For this review, take the finished solid that the model builds, in its own axes (mm). A direction names the side the tool comes from. Round coordinates to 2 decimals unless told otherwise and drop trailing zeros. Order: outer loops, then holes, each group sorted by start corner. A loop starts at its lowest first (then second) coordinate and runs counter-clockwise, first axis right, second up.
from build123d import *

# Parameters (mm, degrees)
SKETCH1_R           = 1.5
BOSS_EXTRUDE1_DEPTH = 2.3
SKETCH2_R           = 5.65
BOSS_EXTRUDE2_DEPTH = 7.7
BOSS_EXTRUDE3_DEPTH = 26.3
SKETCH5_R           = 1
BOSS_EXTRUDE4_DEPTH = 5.5


with BuildPart() as part:
    # Sketch1 → Boss-Extrude1 (new body)
    with BuildSketch(Plane(origin=(0, 0, 0), x_dir=(1, 0, 0), z_dir=(0, 1, 0))):
        with BuildLine():
            Line((-3, 5.765), (3, 5.765))
            Line((3, 5.765), (10.043565082, 3.861472766))
            ThreePointArc((10.043565082, 3.861472766), (13, 0), (10.043565082, -3.861472766))
            Line((10.043565082, -3.861472766), (3, -5.765))
            Line((3, -5.765), (-3, -5.765))
            Line((-3, -5.765), (-10.043565082, -3.861472766))
            ThreePointArc((-10.043565082, -3.861472766), (-13, 0), (-10.043565082, 3.861472766))
            Line((-10.043565082, 3.861472766), (-3, 5.765))
        make_face()
        with Locations((9, 0)):
            Circle(SKETCH1_R, mode=Mode.SUBTRACT)
        with Locations((-9, 0)):
            Circle(SKETCH1_R, mode=Mode.SUBTRACT)
    extrude(amount=-BOSS_EXTRUDE1_DEPTH)

    # Sketch2 → Boss-Extrude2 (add)
    with BuildSketch(Plane.XZ.offset(2.3)):
        Circle(SKETCH2_R)
    extrude(amount=BOSS_EXTRUDE2_DEPTH)

    # Sketch3 → Boss-Extrude3 (add)
    with BuildSketch(Plane.XZ.offset(10)):
        Polygon((-4, 5.765), (4, 5.765), (6.5, 2.765), (6.5, -5.235), (-6.5, -5.235), (-6.5, 2.765), align=None)
    extrude(amount=BOSS_EXTRUDE3_DEPTH)

    # Sketch4 → Cut-Revolve1 (revolve, cut)
    with BuildSketch(Plane.XY):
        Polygon((3.5, -36.3), (10, -29.8), (10, -36.3), align=None)
    revolve(axis=Axis((0, -36.3, 0), (0, 1, 0)), mode=Mode.SUBTRACT)

    # Sketch5 → Boss-Extrude4 (add)
    with BuildSketch(Plane.XZ.offset(36.3)):
        Circle(SKETCH5_R)
    extrude(amount=BOSS_EXTRUDE4_DEPTH)


solid = part.part
(1) Clearance check with flat-ended pins moving along their axes: P1, Ø14.5, axis at x = 0, y = -21, coming from the -Z side (3 decimals); P2, Ø5, axis at y = -29, z = -3.5, coming from the +X side; P3, Ø2.5, axis at y = -17, z = -2.5, coming from the -X side. State where each tip first meets the part, or that it passes through.
(2) Wall thickness on L1, parallel to Z at x = -2.5, y = -22 (3 decimals); L2, parallel to Y at x = -1.75, z = 5.5; L3, parallel to Y at x = -6.75, z = 3: over which ranges is each line inside the solid? List them lowest first.
(3) Add section B-B on x = 0. Give the boundary of the cut face in (y, z) (3 decimals).
(4) Add section C-C on x = 9. Give the boundary of the cut face in (y, z), plus the area to 3 significant figures.
(5) Tool access review of faces 5 (the face through (0, -39, -1)), 6 (the face through (-6.57, -1.13, -4.8)), 7 (the face through (5.23, -21.36, 4.29)): name each direction out of +Z, -Z, +X, -X, +Y, -Y from which nothing blocks a thin tool from reaching the whole face with its end or side.
(6) Add section A-A on z = 0. Give the boundary of the cut face in (x, y).
(7) Draft analysis for pull direction Y (two halves, no side actions). For faces 1 (the face through (0, -41.8, 0)), 2 (the face through (5.39, -6.1, 1.7)), 3 (the face through (-6.5, -21, -1)), 4 (the face through (5, -10, 3)), state which applies: pulls with the +Y half, pulls with the -Y half, needs draft (parallel to the pull), parting line crosses it, or undercut.
(8) Add section D-D on y = -18. Give the boundary of the cut face in (x, z) (3 decimals), plus the area to 4 significant figures.
Here are the results:
1. P1: stops at z = -5.235
1. P2: stops at x = 6.5
1. P3: stops at x = -6.5
2. L1: z = -5.235 to 5.765
2. L2: y = -34.03 to -10, -2.3 to 0
2. L3: y = -2.3 to 0
3. outline: (-41.8, -1) - (-36.3, -1) - (-36.3, -3.5) - (-34.565, -5.235) - (-10, -5.235) - (-10, -5.65) - (-2.3, -5.65) - (-2.3, -5.765) - (0, -5.765) - (0, 5.765) - (-2.3, 5.765) - (-2.3, 5.65) - (-10, 5.65) - (-10, 5.765) - (-34.035, 5.765) - (-36.3, 3.5) - (-36.3, 1) - (-41.8, 1) - close
4. outline: (-2.3, -4.14) - (0, -4.14) - (0, -1.5) - (-2.3, -1.5) - close; (-2.3, 1.5) - (0, 1.5) - (0, 4.14) - (-2.3, 4.14) - close
4. area: 12.2 mm2
5. face 5: -Y
5. face 6: -Z, -X, +Y
5. face 7: +Z, +X, -Y
6. outline: (-13, -2.3) - (-10.5, -2.3) - (-10.5, 0) - (-13, 0) - close; (-7.5, -2.3) - (-5.65, -2.3) - (-5.65, -10) - (-6.5, -10) - (-6.5, -33.3) - (-3.5, -36.3) - (-1, -36.3) - (-1, -41.8) - (1, -41.8) - (1, -36.3) - (3.5, -36.3) - (6.5, -33.3) - (6.5, -10) - (5.65, -10) - (5.65, -2.3) - (7.5, -2.3) - (7.5, 0) - (-7.5, 0) - close; (10.5, -2.3) - (13, -2.3) - (13, 0) - (10.5, 0) - close
7. face 1: pulls with the -Y half
7. face 2: undercut
7. face 3: needs draft
7. face 4: undercut
8. outline: (-6.5, -5.235) - (6.5, -5.235) - (6.5, 2.765) - (4, 5.765) - (-4, 5.765) - (-6.5, 2.765) - close
8. area: 135.5 mm2
